Geometry check sheet. Reference: the model listing, model coordinates, mm. Give positions to 0.01 mm unless a question says otherwise; leave off trailing zeros. Write each loop counter-clockwise with the first axis right and the second up, starting at its lowest first coordinate (ties: lowest second). Pieces come first, ordered by that corner, then holes.
(1) Cross-section at A-A (y = -2.1). Record the boundary of the cut face in (x, z).
(2) Cross-section at C-C (x = 69). Record the boundary of the cut face in (y, z), and give its area (3 significant figures).
(3) Depth check by flat-ended pin: P1, Ø1.5, axis at y = -2.5, z = -78, coming from the +X side; P2, Ø3, axis at y = -4.5, z = -136.5, coming from the +X side; P3, Ø3, axis at x = 35, z = -41, coming from the +Y side. Enter the tip coordinate at first touch or a pass-through.
(4) Cross-section at B-B (z = -141). Record the boundary of the cut face in (x, y), and give its area (3 significant figures).
(5) Thickness scan on line 1 along X through (y, z) = (-0.6, -97); line 2 along X through (y, z) = (-4.1, -36). Record the ranges inside material, lowest first.
```python
from build123d import *

# Parameters (mm, degrees)
F1_DEPTH = 5.842
F2_R     = 6.35
F3_R     = 12.7


# Not quite as in the source:
# - a length typed as a fraction of an inch, garbled in the dataset ("3 / 203.2 mm" for 3/8 in), is restored


with BuildPart() as f1:
    # F0 (on Front) → F1 (new body)
    with BuildSketch(Plane.XZ):
        Polygon((50.8, 0), (0, 0), (55.4690637022, -152.4), (106.2690637022, -152.4), align=None)
    extrude(amount=F1_DEPTH)

    # F2
    f2_edges = [f1.edges().sort_by_distance(p)[0] for p in [
        (55.469064, -2.921, -152.4),
        (50.8, -2.921, 0),
        (0, -2.921, 0),
    ]]
    fillet(f2_edges, radius=F2_R)

    # F3
    f3_edges = [f1.edges().sort_by_distance(p)[0] for p in [
        (106.269064, -2.921, -152.4),
    ]]
    fillet(f3_edges, radius=F3_R)


solid = f1.part
```
Reply:
1. outline: (3.1, -8.52) - (53.95, -148.22) arc R6.35 ccw to (59.92, -152.4) - (88.13, -152.4) arc R12.7 ccw to (100.07, -135.36) - (52.32, -4.18) arc R6.35 ccw to (46.35, 0) - (9.07, 0) arc R6.35 ccw to start
2. outline: (-5.84, -152.4) - (0, -152.4) - (0, -50) - (-5.84, -50) - close
2. area: 598 mm2
3. P1: stops at x = 79.46
3. P2: stops at x = 100.72
3. P3: stops at y = 0
4. outline: (51.32, -5.84) - (100.76, -5.84) - (100.76, 0) - (51.32, 0) - close
4. area: 289 mm2
5. line 1: x = 35.31 to 86.11
5. line 2: x = 13.1 to 63.9
